Design review of the part built by this model. Coordinates are the model's own, in mm. A direction names the side the tool comes from. Give positions to 0.01 mm unless a question says otherwise; leave off trailing zeros. Order: outer loops, then holes, each group sorted by start corner. A loop starts at its lowest first (then second) coordinate and runs counter-clockwise, first axis right, second up. Notation, with made-up numbers: (15.25, 73) -> (24.25, 73) arc R22 ccw to (24.25, 96) -> close; hole circle Ø10 at (68, 68.5). An arc over 180 degrees is marked (long way). One line per item, written item: value. Start each with the question number.
1) Wall thickness on line 1 along Z through (x, y) = (0, 3); line 2 along X through (y, z) = (15, 0); line 3 along X through (y, z) = (3.5, -10): over which ranges is each line inside the solid? List them lowest first. Write a range as from..to.
2) Consider section B-B (x = -18). State the section outline as (y, z) points, plus the area to 3 significant figures.
3) Consider section A-A (z = 20). State the section outline as (x, y) points, plus the area to 3 significant figures.
4) The part is to be moulded in two halves that separate along Z. For faces 1 (the face through (0, 10, 0)), 2 (the face through (2.5, 28, 9)), 3 (the face through (-14.842, 4.93, 9.675)), 4 (the face through (8.3, 34.2, 0.2)), say which applies: released by +Z, released by -Z, zero draft, split by the parting line, or undercut.
5) For pin 1 (5 mm diameter, centred on y = 4.5, z = 4.5, fed in from -X); pin 2 (20 mm diameter, centred on x = 2, z = 1.5, fed in from +Y); pin 3 (8 mm diameter, centred on x = -7.5, z = 19, fed in from +Y); pin 4 (3 mm diameter, centred on x = -17.32, z = 10, fed in from +Y), all flat-tipped, find the tip position at first contact; note any pin that passes through.
6) Consider section D-D (z = -20). State the section outline as (x, y) points.
7) Tool access review of faces 5 (the face through (-9.58, 4.93, 23.09)), 6 (the face through (0, 5, -17)), 7 (the face through (0, 22, -6)), 8 (the face through (2.5, 28, -9)): name each direction out of +Z, -Z, +X, -X, +Y, -Y from which nothing blocks a thin tool from reaching the whole face with its end or side.
8) Consider section C-C (z = 0). State the section outline as (x, y) points, plus the area to 3 significant figures.
from build123d import *

# Parameters (mm, degrees)
SKETCH1_R               = 25
BOSS_EXTRUDE1_DEPTH     = 10
SKETCH1_3_R             = 12.5
SKETCH1_3_R_2           = 6
BOSS_EXTRUDE2_DEPTH     = 35
CUT_EXTRUDE1_START      = 5
CUT_EXTRUDE1_DEPTH      = 5
CUT_EXTRUDE2_DEPTH      = 50.749371855
CUT_EXTRUDE2_DEPTH_BACK = 50.749371855
SKETCH2_W               = 5
SKETCH2_H               = 12
SKETCH3_R               = 2.5
CUT_EXTRUDE3_DEPTH      = 50.749371855
CIRPATTERN1_COUNT       = 6
CHAMFER1_SIZE           = 5


with BuildPart() as part:
    # Sketch1 → Boss-Extrude1 (new body)
    with BuildSketch(Plane(origin=(0, 0, 0), x_dir=(1, 0, 0), z_dir=(0, 1, 0))):
        with Locations(Location((0, 0, 0), (0, 0, 270))):
            Circle(SKETCH1_R)
    extrude(amount=BOSS_EXTRUDE1_DEPTH)

    # Sketch1<3> → Boss-Extrude2 (add)
    with BuildSketch(Plane(origin=(0, 0, 0), x_dir=(1, 0, 0), z_dir=(0, 1, 0))):
        with Locations(Location((0, 0, 0), (0, 0, 270))):
            Circle(SKETCH1_3_R)
        with Locations(Location((0, 0, 0), (0, 0, 270))):
            Circle(SKETCH1_3_R_2, mode=Mode.SUBTRACT)
    extrude(amount=BOSS_EXTRUDE2_DEPTH)

    # Sketch1<5> → Cut-Extrude1 (cut)
    with BuildSketch(Plane(origin=(0, 0, 0), x_dir=(1, 0, 0), z_dir=(0, 1, 0)).offset(CUT_EXTRUDE1_START)):
        with BuildLine():
            ThreePointArc((20, 15), (0, 25), (-20, 15))
            Line((-20, 15), (20, 15))
        make_face()
    extrude(amount=CUT_EXTRUDE1_DEPTH, mode=Mode.SUBTRACT)

    # Sketch2 → Cut-Extrude2 (cut, two sides: drawn at the far end of the back side and taken through both)
    with BuildSketch(Plane.XY.offset(-CUT_EXTRUDE2_DEPTH_BACK)):
        with Locations((0, 29)):
            Rectangle(SKETCH2_W, SKETCH2_H)
    extrude(amount=CUT_EXTRUDE2_DEPTH + CUT_EXTRUDE2_DEPTH_BACK, mode=Mode.SUBTRACT)

    # Sketch3 → Cut-Extrude3 (cut, through all)
    with BuildSketch(Plane(origin=(0, 0, 0), x_dir=(1, 0, 0), z_dir=(0, 1, 0))):
        with Locations(Location((0, 20, 0), (0, 0, 270))):
            Circle(SKETCH3_R)
    cut_extrude3 = extrude(amount=CUT_EXTRUDE3_DEPTH, mode=Mode.SUBTRACT)

    # CirPattern1: Cut-Extrude3 ×6 about axis
    cirpattern1_axis = Axis((0, 0, 0), (0, 1, 0))
    for i in range(1, CIRPATTERN1_COUNT):
        add(cut_extrude3.rotate(cirpattern1_axis, i * 360 / CIRPATTERN1_COUNT), mode=Mode.SUBTRACT)

    # Chamfer1
    chamfer1_edges = [part.edges().sort_by_distance(p)[0] for p in [
        (-12.5, 35, 0),
        (12.5, 35, 0),
    ]]
    chamfer(chamfer1_edges, length=CHAMFER1_SIZE)


solid = part.part
Checked values:
1. line 1: z = -25..-22.5, -17.5..17.5, 22.5..25
1. line 2: x = -12.5..-6, 6..12.5
1. line 3: x = -22.91..-19.82, -14.82..14.82, 19.82..22.91
2. outline: (0, -17.35) -> (5, -17.35) -> (5, -15) -> (10, -15) -> (10, -12.41) -> (0, -12.41) -> close; (0, -7.59) -> (10, -7.59) -> (10, 7.59) -> (0, 7.59) -> close; (0, 12.41) -> (10, 12.41) -> (10, 17.35) -> (0, 17.35) -> close
2. area: 239 mm^2
3. outline: (-15, 0) -> (-2.5, 0) -> (-2.5, 10) -> (-15, 10) -> close; (2.5, 0) -> (15, 0) -> (15, 10) -> (2.5, 10) -> close
3. area: 250 mm^2
4. face 1: undercut
4. face 2: zero draft
4. face 3: undercut
4. face 4: split by the parting line
5. pin 1: stops at x = -24.92
5. pin 2: stops at y = 35
5. pin 3: stops at y = 10
5. pin 4: passes through
6. outline: (-15, 0) -> (-2.5, 0) -> (-2.5, 5) -> (-15, 5) -> close; (2.5, 0) -> (15, 0) -> (15, 5) -> (2.5, 5) -> close
7. face 5: +Y, -Y
7. face 6: -Z, +X, -X, +Y
7. face 7: +Y
7. face 8: +Z, -Z, +Y
8. outline: (-25, 0) -> (25, 0) -> (25, 10) -> (12.5, 10) -> (12.5, 30) -> (7.5, 35) -> (6, 35) -> (6, 10) -> (-6, 10) -> (-6, 35) -> (-7.5, 35) -> (-12.5, 30) -> (-12.5, 10) -> (-25, 10) -> close
8. area: 800 mm^2
